For this review, take the finished solid that the model builds, in its own axes (mm). A direction names the side the tool comes from. Round coordinates to 2 decimals unless told otherwise and drop trailing zeros. Write each loop counter-clockwise with the first axis right and the second up, starting at its lowest first coordinate (ties: lowest second). Pieces come first, ordered by that corner, then holes.
from build123d import *

# Parameters (mm, degrees)
SCHIZZO2_R               = 1.75
TAGLIO_ESTRUSIONE1_DEPTH = 10
SMUSSO1_SIZE             = 0.25
RACCORDO1_R              = 0.25


with BuildPart() as part:
    # Schizzo1 → Rivoluzione1 (revolve)
    with BuildSketch(Plane.XY):
        Polygon((0, 0), (0, 15), (1, 15), (1, 13.5), (7, 13.5), (7, 10), (1, 10), (1, 0), align=None)
    revolve(axis=Axis((-4, 0, 0), (0, 1, 0)))

    # Schizzo2 → Taglio-Estrusione1 (cut)
    with BuildSketch(Plane(origin=(0, 13.5, 0), x_dir=(1, 0, 0), z_dir=(0, 1, 0))):
        with Locations((-4, -8)):
            Circle(SCHIZZO2_R)
        with Locations((-12, 0)):
            Circle(SCHIZZO2_R)
        with Locations((-4, 8)):
            Circle(SCHIZZO2_R)
        with Locations((4, 0)):
            Circle(SCHIZZO2_R)
    extrude(amount=-TAGLIO_ESTRUSIONE1_DEPTH, mode=Mode.SUBTRACT)

    # Smusso1
    smusso1_edges = [part.edges().sort_by_distance(p)[0] for p in [
        (-15, 10, 0),
        (-9, 0, 0),
        (-8, 15, 0),
        (-9, 15, 0),
        (-15, 13.5, 0),
    ]]
    chamfer(smusso1_edges, length=SMUSSO1_SIZE)

    # Raccordo1
    raccordo1_edges = [part.edges().sort_by_distance(p)[0] for p in [
        (-9, 10, 0),
        (-9, 13.5, 0),
    ]]
    fillet(raccordo1_edges, radius=RACCORDO1_R)


solid = part.part
(1) We need section B-B, the plane x = -4. State how many separate pieces and enclosed holes the cut face has, and give its area (3 significant figures).
Geometry check:
separate pieces: 4
enclosed holes: 0
area: 47.2 mm2
(2) For line 1 along Z through (x, y) = (-4, 12.55); line 2 along X through (y, z) = (11.05, 0); line 3 along Y through (x, z) = (-13.25, 2), list the stretches that pass through material, from the lowest coordinate up.
Geometry check:
line 1: z = -11 to -9.75, -6.25 to -4, 4 to 6.25, 9.75 to 11
line 2: x = -15 to -13.75, -10.25 to -8, 0 to 2.25, 5.75 to 7
line 3: y = 10 to 13.5
(3) We need section D-D, the plane y = 3.5. Give the boundary of the cut face in (x, z).
Geometry check:
outline: circle Ø10 at (-4, 0); hole circle Ø8 at (-4, 0)
(4) Mouldability with a two-part tool opening along X and no side actions: class faces 4 (the face through (-5.29, 11.77, -9.18)), 5 (the face through (-8, 0, 2)), 6 (the face through (2.25, 11.77, -0.08)), 7 (the face through (-9, 14, 0)) as pulls with the +X half, pulls with the -X half, needs draft (parallel to the pull), parting line crosses it, or undercut.
Geometry check:
face 4: undercut
face 5: needs draft
face 6: undercut
face 7: parting line crosses it
(5) For pin 1 Ø5.5 at (x, z) = (-12, 0) entering from -Y; pin 2 Ø4.5 at (x, z) = (-4, 8) entering from +Y; pin 3 Ø5 at (y, z) = (6.5, 3) entering from +X, all flat-tipped, find the tip position at first contact; note any pin that passes through.
Geometry check:
pin 1: stops at y = 10
pin 2: stops at y = 13.5
pin 3: stops at x = 0.97
(6) For faces 1 (the face through (-5.75, 11.77, 7.92)), 2 (the face through (-1, 13.5, 5)), 3 (the face through (1, 10, -3)), list the 3-axis set-ups (+Z, -Z, +X, -X, +Y, -Y) from which the entire face can be reached by the end or side of a thin tool; tool diameter is ignored.
Geometry check:
face 1: +Y, -Y
face 2: +Y
face 3: -Y
(7) We need section A-A, the plane y = 11.5. Give the boundary of the cut face in (x, z), and give its area (3 significant figures).
Geometry check:
outline: circle Ø22 at (-4, 0); hole circle Ø3.5 at (-12, 0); hole circle Ø8 at (-4, 0); hole circle Ø3.5 at (-4, -8); hole circle Ø3.5 at (-4, 8); hole circle Ø3.5 at (4, 0)
area: 291 mm2
